```python
from build123d import *

# Parameters (mm, degrees)
F1_DEPTH = 3
F2_W     = 100
F2_H     = 44
F3_DEPTH = 1.5
F4_W     = 105
F4_H     = 2
F5_DEPTH = 26
F6_W     = 6.5
F6_H     = 71.201939
F6_H_2   = 68.703625
F7_DEPTH = 26


with BuildPart() as f1:
    # F0 (on Top) → F1 (new body)
    with BuildSketch(Plane.XY):
        Polygon((9.09921, 26.634615), (-43.40079, 26.634615), (-43.40079, 22.634615), (-53.269234, 22.634615), (-59.40079, 11.346154), (-59.40079, 7.634615), (-54.40079, 7.634615), (-54.40079, 1.634615), (-54.40079, -4.365385), (-59.40079, -4.365385), (-59.40079, -8.076923), (-53.269234, -19.365385), (-43.40079, -19.365385), (-43.40079, -23.365385), (61.59921, -23.365385), (61.59921, -19.365385), (71.467653, -19.365385), (77.59921, -8.076923), (77.59921, -4.365385), (72.59921, -4.365385), (72.59921, 7.634615), (77.59921, 7.634615), (77.59921, 11.346154), (71.467653, 22.634615), (61.59921, 22.634615), (61.59921, 26.634615), align=None)
    extrude(amount=F1_DEPTH)

    # F2 (on face) → F3 (join)
    with BuildSketch(Plane.XY.offset(3)):
        with Locations((9.09921, 1.634615)):
            Rectangle(F2_W, F2_H)
    extrude(amount=F3_DEPTH)

    # F4 (on face) → F5 (join)
    with BuildSketch(Plane(origin=(0, 0, 0), x_dir=(1, 0, 0), z_dir=(0, 0, -1))):
        with Locations((9.09921, 22.365385)):
            Rectangle(F4_W, F4_H)
        with Locations((9.09921, 18.365385)):
            Rectangle(F4_W, F4_H)
        with Locations((9.09921, 14.365385)):
            Rectangle(F4_W, F4_H)
        with Locations((9.09921, 10.365385)):
            Rectangle(F4_W, F4_H)
        with Locations((9.09921, 6.365385)):
            Rectangle(F4_W, F4_H)
        with Locations((9.09921, 2.365385)):
            Rectangle(F4_W, F4_H)
        with Locations((9.09921, -1.634615)):
            Rectangle(F4_W, F4_H)
        with Locations((9.09921, -5.634615)):
            Rectangle(F4_W, F4_H)
        with Locations((9.09921, -9.634615)):
            Rectangle(F4_W, F4_H)
        with Locations((9.09921, -13.634615)):
            Rectangle(F4_W, F4_H)
        with Locations((9.09921, -17.634615)):
            Rectangle(F4_W, F4_H)
        with Locations((9.09921, -21.634615)):
            Rectangle(F4_W, F4_H)
        with Locations((9.09921, -25.634615)):
            Rectangle(F4_W, F4_H)
    extrude(amount=F5_DEPTH)

    # F6 (on face) → F7 (cut)
    with BuildSketch(Plane(origin=(0, 0, -26), x_dir=(1, 0, 0), z_dir=(0, 0, -1))):
        with Locations((-15.15079, -5.566442)):
            Rectangle(F6_W, F6_H)
        with Locations((33.34921, -3.692707)):
            Rectangle(F6_W, F6_H_2)
    extrude(amount=-F7_DEPTH, mode=Mode.SUBTRACT)


solid = f1.part
```
CAD build for the part. Positions are in the model's coordinates, mm. A direction names the side the tool comes from. Round coordinates to 2 decimals unless told otherwise and drop trailing zeros. Write each loop counter-clockwise with the first axis right and the second up, starting at its lowest first coordinate (ties: lowest second). Pieces come first, ordered by that corner, then holes. Notation, with made-up numbers: M -34,1 L 20,1 A26 cw 20,28 Z; hole C 59.25,-35.5 d5. An arc over 180 degrees is marked long. One line per question, with ' | ' between items.
1. Mould opens along Y. For faces 3 (the flat face through (9, 12.635, -13)), 4 (the flat face through (-56.29, 17.07, 1.48)), 5 (the flat face through (77.599, 9, 1)) say: pulls with the +Y half, pulls with the -Y half, needs draft (parallel to the pull), parting line crosses it, or undercut.
Working result:
face 3: undercut | face 4: pulls with the +Y half | face 5: needs draft
2. Cut at A-A on x = -14. Write the cut outline in (y, z).
Working result:
outline: M -23.37,0 L 26.63,0 L 26.63,3 L 23.63,3 L 23.63,4.5 L -20.37,4.5 L -20.37,3 L -23.37,3 Z
3. Which spindle directions (+Z, -Z, +X, -X, +Y, -Y) get a long thin tool onto all of the face, cutting with end or side? Do faces 1 (the flat face through (-31, -19.365, -13)), 2 (the flat face through (61.599, 25, -12)). Say none if no direction does.
Working result:
face 1: -Z, +X, -X | face 2: +Z, -Z, +X, +Y
4. Cut at B-B on z = -11. Count the separate pieces of the cut face and the enclosed holes in it, and give its area (3 significant figures).
Working result:
separate pieces: 39 | enclosed holes: 0 | area: 2,390 mm2
5. Probe L1, parallel to X at y = -3, z = -3.5; L2, parallel to Z at x = -39.5, y = 8.5; L3, parallel to Z at x = 64.5, y = 6. List the from-to ranges inside material, lowest first. Write a range as from..to.
Working result:
L1: -43.4..-18.4, -11.9..30.1, 36.6..61.6 | L2: 0..4.5 | L3: 0..3
6. Pin check, flat tips, straight feed: pin 1 Ø10 at (y, z) = (6, -8.5) entering from +X; pin 2 Ø4.5 at (y, z) = (-20.5, -5.5) entering from -X. Stop position of each tip, or through.
Working result:
pin 1: x = 61.6 | pin 2: x = -43.4
